from build123d import *

# Parameters (mm, degrees)
SKETCH1_R           = 20
BOSS_EXTRUDE1_DEPTH = 15
SKETCH2_W           = 40
SKETCH2_H           = 5
BOSS_EXTRUDE2_DEPTH = 15
SKETCH3_R           = 15.875
CUT_EXTRUDE1_DEPTH  = 10


with BuildPart() as part:
    # Sketch1 → Boss-Extrude1 (new body)
    with BuildSketch(Plane.XY):
        Circle(SKETCH1_R)
    extrude(amount=BOSS_EXTRUDE1_DEPTH)

    # Sketch2 → Boss-Extrude2 (add)
    with BuildSketch(Plane(origin=(0, 0, 0), x_dir=(-1, 0, 0), z_dir=(0, 0, -1))):
        with Locations((0, -17.5)):
            Rectangle(SKETCH2_W, SKETCH2_H)
    extrude(amount=-BOSS_EXTRUDE2_DEPTH)

    # Sketch3 → Cut-Extrude1 (cut)
    with BuildSketch(Plane(origin=(0, 0, 0), x_dir=(-1, 0, 0), z_dir=(0, 0, -1))):
        Circle(SKETCH3_R)
    extrude(amount=-CUT_EXTRUDE1_DEPTH, mode=Mode.SUBTRACT)


solid = part.part
Build history of the part. All positions in model axes, mm. A direction names the side the tool comes from. Coordinates: 2 decimals unless noted, no trailing zeros. Order: outer loops, then holes, each group sorted by start corner. A loop starts at its lowest first (then second) coordinate and runs counter-clockwise, first axis right, second up. Notation, with made-up numbers: M 62,-2.75 L 71,-2.75 A25 ccw 71,30.25 Z; hole C -14,-34.5 d2. An arc over 180 degrees is marked long. One line per question, with ' | ' between items. Start each with the question number.
Q1. Flat gauge pins, fed straight in: pin 1 Ø5 at (x, y) = (9, -4) entering from -Z; pin 2 Ø3.5 at (x, z) = (15.5, 10.5) entering from +Y; pin 3 Ø2 at (y, z) = (-1.5, 2.5) entering from -X. Where does each tip first touch, or does it go through?
Q2. Probe L1, parallel to X at y = 0.5, z = 3; L2, parallel to Y at x = 0, z = 4.5 (3 decimals); L3, parallel to Z at x = -15.5, y = -3. List the from-to ranges inside material, lowest first. Write a range as from..to.
Q3. Saw through at C-C (z = 3). List the corners of the cut face in (x, y) (3 decimals), then the cut area to 3 significant figures.
Q4. Saw through at B-B (x = 16.5). List the corners of the cut face in (y, z).
Q5. 3-axis set-ups, long thin cutter, end or side, ignore diameter. For faces 5 (the face through (17, -15, 7)), 6 (the face through (-17, -15, 7)), 7 (the face through (0, -20, 7)): which of +Z, -Z, +X, -X, +Y, -Y reach the whole face in a straight line?
Q6. Saw through at D-D (z = 14.25). List the corners of the cut face in (x, y), then the cut area to 3 significant figures.
Q7. Saw through at A-A (y = 0). List the corners of the cut face in (x, z) (3 decimals).
Q8. Two-plate mould, pull along X, no slides. Class faces 1 (the face through (3.441, -15.497, 4.93)), 2 (the face through (0, 0, 15)), 3 (the face through (-20, -18, 7)), 4 (the face through (0, 0, 10)): +X half, -X half, draft (parallel to the pull), parting line (faces both ways), or undercut.
Check values:
1) pin 1: stops at z = 10 | pin 2: stops at y = 14.52 | pin 3: stops at x = -19.99
2) L1: x = -19.99..-15.87, 15.87..19.99 | L2: y = -20..-15.875, 15.875..20 | L3: z = 10..15
3) outline: M -20,-20 L 20,-20 L 20,-15 L 13.229,-15 A20 ccw long -13.229,-15 L -20,-15 Z; hole C 0,0 d31.75 | area: 574 mm2
4) outline: M -20,0 L -15,0 L -15,15 L -20,15 Z; M -11.3,0 L 11.3,0 L 11.3,15 L -11.3,15 Z
5) face 5: +Z, -Z, +X | face 6: +Z, -Z, -X | face 7: +Z, -Z, +X, -X, -Y
6) outline: M -20,-20 L 20,-20 L 20,-15 L 13.23,-15 A20 ccw long -13.23,-15 L -20,-15 Z | area: 1,370 mm2
7) outline: M -20,0 L -15.875,0 L -15.875,10 L 15.875,10 L 15.875,0 L 20,0 L 20,15 L -20,15 Z
8) face 1: undercut | face 2: draft | face 3: -X half | face 4: undercut
